```python
from build123d import *

# Parameters (mm, degrees)
F1_DEPTH = 1193.8
F2_DEPTH = 1155.7


with BuildPart() as f1:
    # F0 (on Right) → F1 (new body, symmetric)
    with BuildSketch(Plane.YZ):
        with BuildLine():
            Line((125.7095026749, 1276.35), (130.0834477884, 1320.759410003))
            ThreePointArc((130.0834477884, 1320.759410003), (65.1201645529, 1325.5513896747), (1.1399e-06, 1327.15))
            ThreePointArc((1.1399e-06, 1327.15), (-65.1201634144, 1325.5513897307), (-130.0834477884, 1320.759410003))
            Line((-130.0834477884, 1320.759410003), (-125.7095026749, 1276.35))
            Line((-125.7095026749, 1276.35), (125.7095026749, 1276.35))
        make_face()
    extrude(amount=F1_DEPTH, both=True)

    # F0 (on Right) → F2 (join, symmetric)
    with BuildSketch(Plane.YZ):
        with BuildLine():
            Line((-130.7128659655, 1327.15), (-130.0834477884, 1320.759410003))
            ThreePointArc((-130.0834477884, 1320.759410003), (-65.1201634144, 1325.5513897307), (1.1399e-06, 1327.15))
            Line((1.1399e-06, 1327.15), (-130.7128659655, 1327.15))
        make_face()
        with BuildLine():
            ThreePointArc((1.1399e-06, 1327.15), (65.1201645529, 1325.5513896747), (130.0834477884, 1320.759410003))
            Line((130.0834477884, 1320.759410003), (130.7128659655, 1327.15))
            Line((130.7128659655, 1327.15), (1.1399e-06, 1327.15))
        make_face()
    extrude(amount=F2_DEPTH, both=True)


solid = f1.part
```
Read the model definition and answer for the solid it produces. Units are mm, in the model's axes. A direction names the side the tool comes from. Round coordinates to 2 decimals unless told otherwise and drop trailing zeros. Write each loop counter-clockwise with the first axis right and the second up, starting at its lowest first coordinate (ties: lowest second). Pieces come first, ordered by that corner, then holes. Notation, with made-up numbers: (13, 84.5) -> (20, 84.5) arc R16 cw to (20, 89.5) -> close; hole circle Ø10 at (47.25, 46.5). An arc over 180 degrees is marked (long way). Answer in a Markdown table with one row per item. Add a question column.
1) Consider line 1 (Y direction, x = 451.5, z = 1279); line 2 (Y direction, x = 201, z = 1318). Determine where each line is inside the solid, lowest interval first.
2) Given P1, Ø12, axis at x = 156.5, z = 1313.5, coming from the +Y side; P2, Ø1, axis at x = 423.5, z = 1309, coming from the +Y side; P3, Ø8, axis at x = 697.5, z = 1317, coming from the +Y side, each flat-ended and moving along its own axis, determine where each tip first touches the part or whether it passes through.
3) Find section B-B, the plane z = 1300.5. Determine the outline of the cut face in (x, y), and give its area (3 significant figures).
4) Find section A-A, the plane x = 938.5. Determine the outline of the cut face in (y, z).
5) Which of the six approach directions +Z, -Z, +X, -X, +Y, -Y give full straight-line access (tool end or side, diameter ignored) to faces 1 (the face through (1175.02, 1.82, 1327.15)), 2 (the face through (-1174.48, 1.82, 1327.15)), 3 (the face through (16, 2, 1327.15))?
Findings below:
| question | item | result |
|---|---|---|
| 1 | line 1 | -125.97 to 125.97 |
| 1 | line 2 | -129.81 to 129.81 |
| 2 | P1 | y = 129.96 |
| 2 | P2 | y = 128.97 |
| 2 | P3 | y = 130.11 |
| 3 | outline | (-1193.8, -128.09) -> (1193.8, -128.09) -> (1193.8, 128.09) -> (-1193.8, 128.09) -> close |
| 3 | area | 612,000 mm² |
| 4 | outline | (-130.71, 1327.15) -> (-125.71, 1276.35) -> (125.71, 1276.35) -> (130.71, 1327.15) -> close |
| 5 | face 1 | +Z, +X |
| 5 | face 2 | +Z, -X |
| 5 | face 3 | +Z, +X, -X, +Y, -Y |
